Autodesk Fusion 360 part; units mm, degrees
sketch "Sketch1" plane through (0, 0, 0) normal (0, 1, 0) x (1, 0, 0)
  line L0 (0, 0) -> (40, 0)
  line L1 (40, 0) -> (40, -16)
  line L2 (40, -16) -> (0, -16)
  line L3 (0, -16) -> (0, 0)
  line L4 (0, -16) -> (40, -16)
  line L5 (40, -16) -> (40, -20)
  line L6 (40, -20) -> (0, -20)
  line L7 (0, -20) -> (0, -16)
  dimension "d1" = 16
  dimension "d2" = 40
  dimension "d3" = 4
extrude "Extrude1" add sketch "Sketch1" along normal blind 4 makes body 1
extrude "Extrude2" add sketch "Sketch1" against normal blind 8 contours L2 L4 L5 L6 L7 bodies 1
sketch "Sketch2" plane through (0, 0, 0) normal (-1, 0, 0) x (0, 0, 1)
  line L0 (20, -8) -> (20, 4)
  line L1 (20, 4) -> (0, 4)
  line L2 (0, 4) -> (0, 0)
  line L3 (0, 0) -> (16, 0)
  line L4 (16, 0) -> (16, -8)
  line L5 (16, -8) -> (20, -8)
sketch "Sketch3" plane through (0, 0, 20) normal (0, 0, 1) x (1, 0, 0)
  line L0 (40, -8) -> (40, 4)
  line L1 (40, 4) -> (0, 4)
  line L2 (0, 4) -> (0, -8)
  line L3 (0, -8) -> (40, -8)
  line L4 (0, -8) -> (40, -8)
  line L5 (0, 4) -> (0, -8)
  line L6 (0, 0) -> (0, -8)
  line L7 (40, 0) -> (40, -8)
  line L8 (40, -4) -> (0, -4)
  line L9 (40, -4) -> (20, -4)
  line L10 (20, -4) -> (0, -4)
  line L11 (0, -4) -> (10, -4)
  line L12 (40, -4) -> (30, -4)
  line L13 (40, -4) -> (20, -4)
  circle A0 centre (20, -4) radius 3
  circle A1 centre (20, -4) radius 1.5
  circle A2 centre (30, -4) radius 3
  circle A3 centre (30, -4) radius 1.5
  circle A4 centre (10, -4) radius 3
  circle A5 centre (10, -4) radius 1.5
  point P0 (40, 0)
  dimension "d8" = 20
  dimension "d9" = 6
  dimension "d10" = 3
  dimension "d11" = 6
  dimension "d12" = 3
  dimension "d13" = 6
  dimension "d14" = 3
extrude "Extrude3" cut sketch "Sketch3" against normal blind 4 contours L8 L9 L12 L13 A3 | L8 L9 L12 L13 A3 bodies 1
extrude "Extrude4" cut sketch "Sketch3" against normal blind 4 contours L8 L9 L10 L13 A1 | L8 L9 L10 L13 A1 bodies 1
extrude "Extrude5" cut sketch "Sketch3" against normal blind 4 contours L8 L10 L11 A5 | L8 L10 L11 A5 bodies 1
extrude "Extrude6" cut sketch "Sketch3" against normal blind 2 contours L8 L9 L12 L13 A2 A3 | L8 L9 L12 L13 A2 A3 | L8 L10 L11 A4 A5 | L8 L10 L11 A4 A5 | L8 L9 L10 L13 A0 A1 | L8 L9 L10 L13 A0 A1 bodies 1
sketch "Sketch4" plane through (0, 0, 0) normal (0, -1, 0) x (1, 0, 0)
  line L0 (40, 16) -> (0, 16)
  line L1 (0, 16) -> (0, 0)
  line L2 (0, 0) -> (40, 0)
  line L3 (40, 0) -> (40, 16)
  line L4 (0, 0) -> (0, 8)
  line L5 (0, 8) -> (40, 8)
  line L6 (0, 8) -> (20, 8)
  line L7 (20, 8) -> (40, 8)
  circle A0 centre (10, 8) radius 3
  circle A1 centre (20, 8) radius 3
  circle A2 centre (30, 8) radius 3
  circle A3 centre (10, 8) radius 1.5
  circle A4 centre (20, 8) radius 1.5
  circle A5 centre (30, 8) radius 1.5
  dimension "d23" = 8
  dimension "d24" = 6
  dimension "d25" = 6
  dimension "d26" = 6
  dimension "d27" = 3
  dimension "d28" = 3
  dimension "d29" = 3
extrude "Extrude7" cut sketch "Sketch4" against normal blind 2 contours L5 L7 A2 A5 | L5 L7 A2 A5 | L5 L6 A0 A3 | L5 L6 A0 A3 | L5 L6 L7 A1 A4 | L5 L6 L7 A1 A4 bodies 1
extrude "Extrude8" cut 3 faces at (30.1453, 0, 7.036) (20.1453, 0, 7.036) (10.5866, 0, 7.6267) along direction (0, 1, 0) blind 30 on bodies 1 bodies 1
mirror "Mirror1" about plane through (0, 0, 0) normal (0, 0, -1) of bodies 1 makes body 2
move_body "Move1" bodies 1 to x (1, 0, 0) y (0, 1, 0) z (0, 0, 1) at (0, 0, -20)
sketch "Sketch5" plane through (0, 0, -4) normal (0, 0, -1) x (-1, 0, 0)
  circle A0 centre (-10, -4) radius 1.5
  circle A1 centre (-20, -4) radius 1.5
  circle A2 centre (-30, -4) radius 1.5
  line L0 (0, 0) -> (-40, 0)
  line L1 (-40, 0) -> (-40, -8)
  line L2 (-40, -8) -> (0, -8)
  line L3 (0, -8) -> (0, 0)
sketch "Sketch6" plane through (0, 0, 0) normal (-1, 0, 0) x (0, 0, 1)
  line L0 (0, -8) -> (0, 4)
  line L1 (0, 4) -> (-20, 4)
  line L2 (-20, 4) -> (-20, 0)
  line L3 (-20, 0) -> (-4, 0)
  line L4 (-4, 0) -> (-4, -8)
  line L5 (-4, -8) -> (0, -8)
  point P0 (-16, 0)
move_body "Move2" bodies 1 to x (1, 0, 0) y (0, 1, 0) z (0, 0, 1) at (0, 0, 4)
combine "Combine1" operation add target body 2 tool bodies 1
equation "d23 = 16 mm / 2"
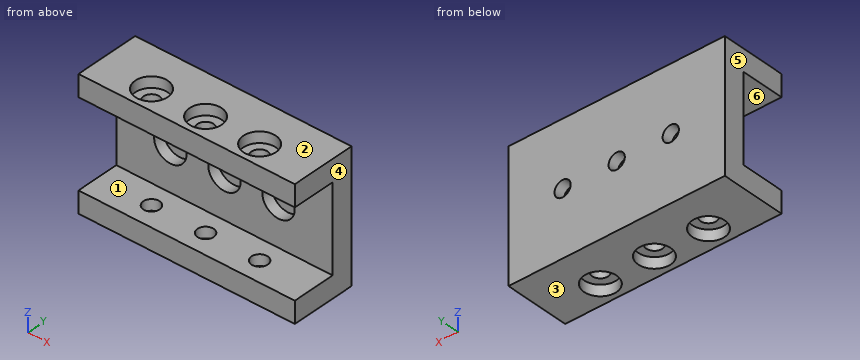
The model under review builds one solid part; all positions refer to its coordinate system, in mm. Face numbers are marked on the shaded views. A direction names the side the tool comes from. Round coordinates to 2 decimals unless told otherwise and drop trailing zeros. Order: outer loops, then holes, each group sorted by start corner. A loop starts at its lowest first (then second) coordinate and runs counter-clockwise, first axis right, second up.
(1) Take a section at A-A, the plane x = 10. Count the separate pieces of the cut face and the enclosed holes in it, plus the area to 3 significant figures.
Working result:
separate pieces: 4
enclosed holes: 0
area: 106 mm2
(2) Mouldability with a two-part tool opening along Z and no side actions: class the marked faces 1, 2, 3 and 4 as released by +Z, released by -Z, zero draft, split by the parting line, or undercut.
Working result:
face 1: undercut
face 2: released by +Z
face 3: released by -Z
face 4: zero draft
(3) Wall thickness on L1, parallel to X at y = 3.1, z = -8; L2, parallel to X at y = -4, z = -19; L3, parallel to Z at x = 22.5, y = -1.25: over which ranges is each line inside the solid? List them lowest first.
Working result:
L1: x = 0 to 8.5, 11.5 to 18.5, 21.5 to 28.5, 31.5 to 40
L2: x = 0 to 7, 13 to 17, 23 to 27, 33 to 40
L3: z = -20 to -16, 0 to 4
(4) Take a section at B-B, the plane z = -8. State the section outline as (x, y) points.
Working result:
outline: (0, 0) - (7, 0) - (7, 2) - (8.5, 2) - (8.5, 4) - (0, 4) - close; (11.5, 2) - (13, 2) - (13, 0) - (17, 0) - (17, 2) - (18.5, 2) - (18.5, 4) - (11.5, 4) - close; (21.5, 2) - (23, 2) - (23, 0) - (27, 0) - (27, 2) - (28.5, 2) - (28.5, 4) - (21.5, 4) - close; (31.5, 2) - (33, 2) - (33, 0) - (40, 0) - (40, 4) - (31.5, 4) - close
(5) Take a section at D-D, the plane x = 37.5. State the section outline as (y, z) points.
Working result:
outline: (-8, -20) - (4, -20) - (4, 4) - (-8, 4) - (-8, 0) - (0, 0) - (0, -16) - (-8, -16) - close
(6) Tool access review of the marked faces 5 and 6: name each direction out of +Z, -Z, +X, -X, +Y, -Y from which nothing blocks a thin tool from reaching the whole face with its end or side.
Working result:
face 5: +Z, -Z, -X, +Y, -Y
face 6: +X, -X, -Y
(7) For P1, Ø5, axis at x = 10, y = -4, coming from the -Z side; P2, Ø9.5, axis at x = 10, z = -8, coming from the -Y side; P3, Ø4, axis at x = 30, z = -8, coming from the -Y side; P4, Ø2.5, axis at x = 20, y = -4, coming from the -Z side, all flat-tipped, find the tip position at first contact; note any pin that passes through.
Working result:
P1: stops at z = -18
P2: stops at y = 0
P3: stops at y = 2
P4: passes through
